Could you check a few things on this model? Use its own coordinates, in mm. A direction names the side the tool comes from. Round coordinates to 2 decimals unless told otherwise and drop trailing zeros. Write each loop counter-clockwise with the first axis right and the second up, starting at its lowest first coordinate (ties: lowest second). Pieces come first, ordered by that corner, then holes. Notation, with made-up numbers: (72.25, 30) - (88.25, 30) arc R12 ccw to (88.25, 49) - close; hole circle Ø11 at (7.25, 45.25). An arc over 180 degrees is marked (long way). Write each question's results on one line, items separated by ' | '. Start each with the question number.
(1) Please list where these lines run through material, in increasing order: line 1 (Y direction, x = 1.9, z = 7.5) (3 decimals); line 2 (Z direction, x = 2.45, y = 41.4) (3 decimals); line 3 (X direction, y = 59.5, z = 12.25). Write a range as [from, to].
(2) Imagine slicing it at B-B on y = 18. Write out the boundary of the cut face in (x, z), then the cut area to 3 significant figures.
(3) Thinking about a two-plate mould opening in Z: for faces 1 (the flat face through (11, 60, 5)), 2 (the flat face through (17, 51, 0)), 3 (the cylindrical face through (1.945, 8.177, 7.58)), 4 (the flat face through (19, 49.9, 8)), which applies, +Z half, -Z half, draft (parallel to the pull), parting line (faces both ways), or undercut?
(4) Imagine slicing it at C-C on x = 23. Write out the boundary of the cut face in (y, z), then the cut area to 3 significant figures.
(5) For P1, Ø4.5, axis at y = 41.4, z = 7.5, coming from the +X side; P2, Ø4.5, axis at x = 23, z = 7, coming from the -Y side; P3, Ø5, axis at y = 8, z = 5.5, coming from the +X side, each with a flat end and sliding along its axis, tell me the tip position at first contact or that it passes through.
(6) Imagine slicing it at D-D on z = 13.25. State how many separate pieces and enclosed holes the cut face has, then the cut area to 3 significant figures.
(7) Imagine slicing it at A-A on x = 37.5. Write out the boundary of the cut face in (y, z), then the cut area to 3 significant figures.
(8) On a 3-axis mill with a long thin cutter (end or side, diameter ignored), from which of +Z, -Z, +X, -X, +Y, -Y can I reach the whole of each face in a straight line? I mean faces 5 (the cylindrical face through (10.92, 4.94, 4.7)), 6 (the flat face through (-1, 60, 13)), 7 (the cylindrical face through (34.3, 40, 10.36)), 8 (the cylindrical face through (1.95, 43.14, 8.05)), 9 (the cylindrical face through (7.716, 4.304, 7.605)). Say none if no direction works.
```python
from build123d import *

# Parameters (mm, degrees)
P_IDAT_VYSUNUT_M1_DEPTH  = 15
SKICA2_R                 = 4.1
ODEBRAT_VYSUNUT_M1_DEPTH = 88.321245983
SKICA3_R                 = 4.05
ODEBRAT_VYSUNUT_M2_DEPTH = 10
ODEBRAT_VYSUNUT_M3_DEPTH = 88.321245983
P_IDAT_VYSUNUT_M2_DEPTH  = 70
SKICA6_W                 = 3.385621722
SKICA6_H                 = 7.5
ODEBRAT_VYSUNUT_M4_DEPTH = 10
SKICA8_W                 = 8
SKICA8_H                 = 44.48438966
ODEBRAT_VYSUNUT_M5_DEPTH = 88.290898193
ZAOBLIT1_R               = 4
SKICA9_R                 = 1.825
ODEBRAT_VYSUNUT_M6_DEPTH = 86.094065598
ZAOBLIT3_R               = 6
ZKOSEN_1_SIZE            = 2


with BuildPart() as part:
    # Skica1 → Přidat vysunutím1 (new body)
    with BuildSketch(Plane.XY):
        Polygon((0, 0), (10, 0), (50, 60), (50, 70), (0, 70), align=None)
    extrude(amount=P_IDAT_VYSUNUT_M1_DEPTH)

    # Skica2 → Odebrat vysunutím1 (cut, through all)
    with BuildSketch(Plane.XY.offset(15)):
        with Locations((35, 60)):
            Circle(SKICA2_R)
    extrude(amount=-ODEBRAT_VYSUNUT_M1_DEPTH, mode=Mode.SUBTRACT)

    # Skica3 → Odebrat vysunutím2 (cut)
    with BuildSketch(Plane.XY.offset(15)):
        with Locations((11, 60)):
            Circle(SKICA3_R)
    extrude(amount=-ODEBRAT_VYSUNUT_M2_DEPTH, mode=Mode.SUBTRACT)

    # Skica4 → Odebrat vysunutím3 (cut, through all)
    with BuildSketch(Plane.XY.offset(15)):
        with BuildLine():
            Line((9, 49.9), (29.116679507, 49.9))
            ThreePointArc((29.116679507, 49.9), (33.525052501, 47.259289628), (33.276930979, 42.126499019))
            Line((33.276930979, 42.126499019), (8.601431306, 5.113249509))
            ThreePointArc((8.601431306, 5.113249509), (7.700950384, 4.295813503), (6.52130557, 4))
            Line((6.52130557, 4), (6.5, 4))
            ThreePointArc((6.5, 4), (4.732233047, 4.732233047), (4, 6.5))
            Line((4, 6.5), (4, 44.9))
            ThreePointArc((4, 44.9), (5.464466094, 48.435533906), (9, 49.9))
        make_face()
    extrude(amount=-ODEBRAT_VYSUNUT_M3_DEPTH, mode=Mode.SUBTRACT)

    # Skica5 → Přidat vysunutím2 (add)
    with BuildSketch(Plane(origin=(0, 70, 0), x_dir=(1, 0, 0), z_dir=(0, 1, 0))):
        with BuildLine():
            Line((-3.385621722, 0), (3, 0))
            Line((3, 0), (3, -15))
            Line((3, -15), (-3.385621722, -15))
            ThreePointArc((-3.385621722, -15), (0, -7.5), (-3.385621722, 0))
        make_face()
    extrude(amount=-P_IDAT_VYSUNUT_M2_DEPTH)

    # Skica6 → Odebrat vysunutím4 (cut)
    with BuildSketch(Plane(origin=(0, 70, 0), x_dir=(1, 0, 0), z_dir=(0, 1, 0))):
        with Locations((-1.692810861, -11.25)):
            Rectangle(SKICA6_W, SKICA6_H)
    extrude(amount=-ODEBRAT_VYSUNUT_M4_DEPTH, mode=Mode.SUBTRACT)

    # Skica8 → Odebrat vysunutím5 (cut, through all)
    with BuildSketch(Plane(origin=(3.594875746, -2.39658383, 0), x_dir=(0, 0, 1), z_dir=(-0.8320502943378438, 0.5547001962252291, 0))):
        with Locations((7.5, 31.267891222)):
            Rectangle(SKICA8_W, SKICA8_H)
    extrude(amount=-ODEBRAT_VYSUNUT_M5_DEPTH, mode=Mode.SUBTRACT)

    # Zaoblit1
    zaoblit1_edges = [part.edges().sort_by_distance(p)[0] for p in [
        (34.941031567, 41.017098626, 3.5),
        (34.941031567, 41.017098626, 11.5),
        (10.265531894, 4.003849117, 11.5),
        (10.265531894, 4.003849117, 3.5),
    ]]
    fillet(zaoblit1_edges, radius=ZAOBLIT1_R - 0.0001)  # a hair under: the kernel refuses the full size

    # Skica9 → Odebrat vysunutím6 (cut, through all)
    with BuildSketch(Plane(origin=(4, 0, 0), x_dir=(0, 0, -1), z_dir=(1, 0, 0))):
        with Locations(Location((-7.5, 10, 0), (0, 0, 90))):
            Circle(SKICA9_R)
        with Locations(Location((-7.5, 41.4, 0), (0, 0, 90))):
            Circle(SKICA9_R)
    extrude(amount=-ODEBRAT_VYSUNUT_M6_DEPTH, mode=Mode.SUBTRACT)

    # Zaoblit3
    zaoblit3_edges = [part.edges().sort_by_distance(p)[0] for p in [
        (10, 0, 7.5),
    ]]
    fillet(zaoblit3_edges, radius=ZAOBLIT3_R)

    # Zkosení1
    zkosen_1_edges = [part.edges().sort_by_distance(p)[0] for p in [
        (50, 70, 7.5),
    ]]
    chamfer(zkosen_1_edges, length=ZKOSEN_1_SIZE)


solid = part.part
```
Response:
1) line 1: [0, 8.175], [11.825, 39.575], [43.225, 70] | line 2: [0, 5.675], [9.325, 15] | line 3: [-1.2, 6.98], [15.02, 30.93], [39.07, 49.67]
2) outline: (-3.39, 0) - (4, 0) - (4, 15) - (-3.39, 15) arc R10 cw to start; (17.19, 0) - (22, 0) - (22, 3.5) - (17.19, 3.5) - close; (17.19, 11.5) - (22, 11.5) - (22, 15) - (17.19, 15) - close | area: 109 mm²
3) face 1: +Z half | face 2: -Z half | face 3: undercut | face 4: draft
4) outline: (19.5, 0) - (26.71, 0) - (26.71, 3.5) - (19.5, 3.5) - close; (19.5, 11.5) - (26.71, 11.5) - (26.71, 15) - (19.5, 15) - close; (49.9, 0) - (70, 0) - (70, 15) - (49.9, 15) - close | area: 352 mm²
5) P1: x = 39.1 | P2: y = 49.9 | P3: x = 16.33
6) separate pieces: 1 | enclosed holes: 3 | area: 1,450 mm²
7) outline: (41.25, 0) - (56.75, 0) - (56.75, 15) - (41.25, 15) - close; (63.25, 0) - (70, 0) - (70, 15) - (63.25, 15) - close | area: 334 mm²
8) face 5: +X | face 6: +Z, -X, +Y | face 7: -Y | face 8: -X | face 9: +Z, -Z
